```python
from build123d import *

# Parameters (mm, degrees)
SKETCH1_R           = 1.6
BOSS_EXTRUDE1_DEPTH = 5
SKETCH2_R           = 3
CUT_EXTRUDE1_DEPTH  = 3


with BuildPart() as part:
    # Sketch1 → Boss-Extrude1 (new body)
    with BuildSketch(Plane.XY.offset(22)):
        with BuildLine():
            Line((0, 4), (15, 4))
            ThreePointArc((15, 4), (19, 0), (15, -4))
            Line((15, -4), (7, -4))
            ThreePointArc((7, -4), (3.5, -7.5), (0, -4))
            ThreePointArc((0, -4), (-4, 0), (0, 4))
        make_face()
        Circle(SKETCH1_R, mode=Mode.SUBTRACT)
        with Locations((15, 0)):
            Circle(SKETCH1_R, mode=Mode.SUBTRACT)
    extrude(amount=BOSS_EXTRUDE1_DEPTH)

    # Sketch2 → Cut-Extrude1 (cut)
    with BuildSketch(Plane.XY.offset(27)):
        Circle(SKETCH2_R)
        with Locations((15, 0)):
            Circle(SKETCH2_R)
    extrude(amount=-CUT_EXTRUDE1_DEPTH, mode=Mode.SUBTRACT)


solid = part.part
```
CAD build for the part. Positions are in the model's coordinates, mm. A direction names the side the tool comes from. Round coordinates to 2 decimals unless told otherwise and drop trailing zeros. Loops run counter-clockwise (first coordinate to the right, second up) from the corner with the lowest first, then second, coordinate; pieces in that order, holes last. Notation, with made-up numbers: M 86.25,50.25 L 93.25,50.25 A19 ccw 93.25,70.25 Z; hole C -38,55 d9. An arc over 180 degrees is marked long. Return JSON: item names as keys, results as strings. Group by question number.
(1) Saw through at A-A, the plane y = 0. List the corners of the cut face in (x, z), and give its area (3 significant figures).
(2) Drop flat-ended pins along their axis: P1, Ø5, axis at x = 15, y = 0, coming from the -Z side; P2, Ø2, axis at x = 0, z = 22.5, coming from the -Y side; P3, Ø3.5, axis at x = 15, y = 0, coming from the +Z side; P4, Ø3, axis at y = -3.5, z = 25, coming from the +X side. Give the stop position or say it passes through.
(3) Tool access for faces 1 (the cylindrical face through (-4, 0, 24)), 2 (the flat face through (16.3, -1.3, 24)): list every direction of +Z, -Z, +X, -X, +Y, -Y with a clear straight run to the whole face (end or side of a thin tool).
(4) Saw through at B-B, the plane x = 0.5. List the corners of the cut face in (y, z), and give its area (3 significant figures).
(5) Saw through at C-C, the plane z = 22.7. List the corners of the cut face in (x, y).
(6) Mould opens along Y. For faces 3 (the flat face through (7, 4, 24)), 4 (the flat face through (11, -4, 24)), 5 (the cylindrical face through (19, 0, 24)), 6 (the cylindrical face through (12, 0, 26)) say: +Y half, -Y half, draft (parallel to the pull), parting line (faces both ways), or undercut.
(7) Saw through at D-D, the plane y = 2.5. List the corners of the cut face in (x, z).
(8) Wall check: probe 1 along X at (y, z) = (0, 23.05); probe 2 along X at (y, z) = (2.5, 26.05); probe 3 along Z at (x, y) = (12.75, -1). Give the ranges that are in metal, low to high. Write a range as [from, to].
Answer list:
{
 "1": {"outline": "M -4,22 L -1.6,22 L -1.6,24 L -3,24 L -3,27 L -4,27 Z; M 1.6,22 L 13.4,22 L 13.4,24 L 12,24 L 12,27 L 3,27 L 3,24 L 1.6,24 Z; M 16.6,22 L 19,22 L 19,27 L 18,27 L 18,24 L 16.6,24 Z", "area": "66.2 mm2"},
 "2": {"P1": "z = 22", "P2": "y = -6.45", "P3": "z = 24", "P4": "x = 18.46"},
 "3": {"face 1": "+Z, -Z, -X", "face 2": "+Z"},
 "4": {"outline": "M -5.8,22 L -1.52,22 L -1.52,24 L -2.96,24 L -2.96,27 L -5.8,27 Z; M 1.52,22 L 4,22 L 4,27 L 2.96,27 L 2.96,24 L 1.52,24 Z", "area": "25.2 mm2"},
 "5": {"outline": "M 0,-4 A3.5 ccw 7,-4 L 15,-4 A4 ccw 15,4 L 0,4 A4 ccw Z; hole C 0,0 d3.2; hole C 15,0 d3.2"},
 "6": {"face 3": "+Y half", "face 4": "-Y half", "face 5": "parting line", "face 6": "undercut"},
 "7": {"outline": "M -3.12,22 L 18.12,22 L 18.12,27 L 16.66,27 L 16.66,24 L 13.34,24 L 13.34,27 L 1.66,27 L 1.66,24 L -1.66,24 L -1.66,27 L -3.12,27 Z"},
 "8": {"probe 1": "[-4, -1.6], [1.6, 13.4], [16.6, 19]", "probe 2": "[-3.12, -1.66], [1.66, 13.34], [16.66, 18.12]", "probe 3": "[22, 24]"}
}
